Read the model definition and answer for the solid it produces. Units are mm, in the model's axes. Coordinates: 2 decimals unless noted, no trailing zeros. Write each loop counter-clockwise with the first axis right and the second up, starting at its lowest first coordinate (ties: lowest second). Pieces come first, ordered by that corner, then holes. Notation, with made-up numbers: (-36.5, 0.25) -> (11.5, 0.25) arc R21 ccw to (11.5, 18.25) -> close; hole circle Ø1 at (74.25, 25.5). An arc over 180 degrees is marked (long way). Answer as a JSON object with one key per item and string values. Group by question number.
(1) Find section D-D (z = -10.5). Give the vertices of the cut face in (x, y).
(2) Find section A-A (z = -18.75). Give the vertices of the cut face in (x, y), then the cut area to 3 significant figures.
(3) Find section C-C (y = 2.2). Count the separate pieces of the cut face and the enclosed holes in it, then the cut area to 3 significant figures.
(4) Straight lines are drawn through the part: L1, parallel to X at y = 1.75, z = -12; L2, parallel to Z at x = -3.32, y = 1.9; L3, parallel to X at y = 1.4, z = -31.25. For each, find the intervals that lie inside material, in ascending order.
(5) Find section B-B (x = -3.32). Give the vertices of the cut face in (y, z).
from build123d import *

# Parameters (mm, degrees)
SKETCH1_W             = 56.64
SKETCH1_H             = 36
BOSS_EXTRUDE1_DEPTH   = 3
F_6_CLEARANCE_HOLE2_D = 3.7973
SKETCH7_W             = 5
SKETCH7_H             = 3
CUT_EXTRUDE1_DEPTH    = 10
FILLET1_R             = 2


with BuildPart() as part:
    # Sketch1 → Boss-Extrude1 (new body)
    with BuildSketch(Plane(origin=(0, 0, 0), x_dir=(1, 0, 0), z_dir=(0, 1, 0))):
        with Locations((-28.32, 18)):
            Rectangle(SKETCH1_W, SKETCH1_H)
    extrude(amount=BOSS_EXTRUDE1_DEPTH)

    # #6 Clearance Hole2 (through all)
    with Locations(Plane(origin=(0, 3, 0), x_dir=(1, 0, 0), z_dir=(0, 1, 0))):
        with Locations((-53.32, 31.25), (-53.32, 18.75), (-53.32, 3.75), (-3.32, 31.25), (-3.32, 18.75), (-3.32, 3.75)):
            Hole(F_6_CLEARANCE_HOLE2_D / 2)

    # Sketch7 → Cut-Extrude1 (cut)
    with BuildSketch(Plane(origin=(0, 3, 0), x_dir=(1, 0, 0), z_dir=(0, 1, 0))):
        with Locations((-52.64, 10.97)):
            Rectangle(SKETCH7_W, SKETCH7_H)
        with Locations((-4, 10.97)):
            Rectangle(SKETCH7_W, SKETCH7_H)
    extrude(amount=-CUT_EXTRUDE1_DEPTH, mode=Mode.SUBTRACT)

    # Fillet1
    fillet1_edges = [part.edges().sort_by_distance(p)[0] for p in [
        (0, 1.5, 0),
        (-56.64, 1.5, 0),
        (-56.64, 1.5, -36),
        (0, 1.5, -36),
    ]]
    fillet(fillet1_edges, radius=FILLET1_R)


solid = part.part
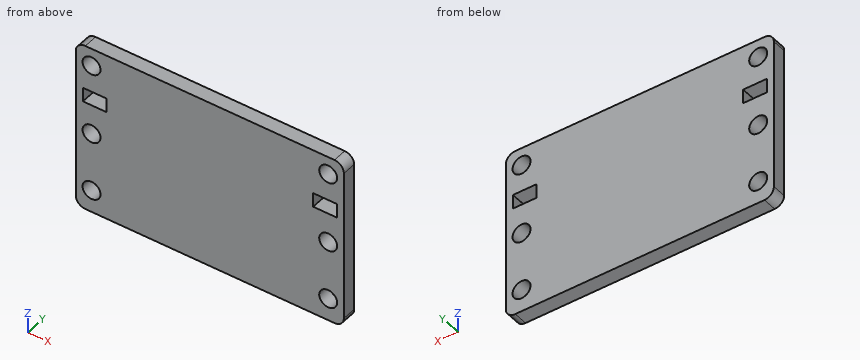
Results below:
{
 "1": {"outline": "(-56.64, 0) -> (-55.14, 0) -> (-55.14, 3) -> (-56.64, 3) -> close; (-50.14, 0) -> (-6.5, 0) -> (-6.5, 3) -> (-50.14, 3) -> close; (-1.5, 0) -> (0, 0) -> (0, 3) -> (-1.5, 3) -> close"},
 "2": {"outline": "(-56.64, 0) -> (-55.22, 0) -> (-55.22, 3) -> (-56.64, 3) -> close; (-51.42, 0) -> (-5.22, 0) -> (-5.22, 3) -> (-51.42, 3) -> close; (-1.42, 0) -> (0, 0) -> (0, 3) -> (-1.42, 3) -> close", "area": "147 mm2"},
 "3": {"separate pieces": "1", "enclosed holes": "8", "area": "1,940 mm2"},
 "4": {"L1": "x = -56.64 to -55.14, -50.14 to -6.5, -1.5 to 0", "L2": "z = -36 to -33.15, -29.35 to -20.65, -16.85 to -12.47, -9.47 to -5.65, -1.85 to 0", "L3": "x = -56.64 to -55.22, -51.42 to -5.22, -1.42 to 0"},
 "5": {"outline": "(0, -36) -> (3, -36) -> (3, -33.15) -> (0, -33.15) -> close; (0, -29.35) -> (3, -29.35) -> (3, -20.65) -> (0, -20.65) -> close; (0, -16.85) -> (3, -16.85) -> (3, -12.47) -> (0, -12.47) -> close; (0, -9.47) -> (3, -9.47) -> (3, -5.65) -> (0, -5.65) -> close; (0, -1.85) -> (3, -1.85) -> (3, 0) -> (0, 0) -> close"}
}
